Autodesk Inventor part; units mm, degrees
ref_plane "YZ Plane" through (0, 0, 0) normal (1, 0, 0) x (0, 1, 0)
ref_plane "XY Plane" through (0, 0, 0) normal (0, 0, 1) x (1, 0, 0)
ref_plane "Work Plane1" through (0, 0, -11) normal (0, 0, -1) x (-1, 0, 0)
sketch "Sketch1" plane through (0, 0, 0) normal (0, 0, 1) x (1, 0, 0)
  circle A0 centre (0, 0) radius 32
  dimension "d0" = 64
extrude "Extrusion1" add sketch "Sketch1" along normal blind 10
sketch "Sketch2" plane through (0, 0, 10) normal (0, 0, 1) x (1, 0, 0)
  circle A0 centre (0, 0) radius 32
  line L0 (-31.4325, 6) -> (-6, 6)
  line L1 (-6, 6) -> (-6, 31.4325)
  dimension "d3" = 6
extrude "Extrusion2" cut sketch "Sketch2" against normal through all contours L1 L0 A0 picked at (-8.4207, 22.185)
pattern_circular "Circular Pattern1" count 4 over 360 about axis through (0, 0, 0) along (0, 0, 1) of "Extrusion2"
sketch "Sketch3" plane through (0, 0, 10) normal (0, 0, 1) x (1, 0, 0)
  arc A0 (-31.4325, 6) -> (-31.4325, -6) centre (0, 0) ccw
  arc A1 (31.4325, -6) -> (31.4325, 6) centre (0, 0) ccw
  line L0 (-31.749, 4) -> (31.749, 4)
  line L1 (-31.749, -4) -> (31.749, -4)
  dimension "d9" = 8
extrude "Extrusion3" cut sketch "Sketch3" against normal blind 8
pattern_circular "Circular Pattern2" count 2 over 90 about axis through (0, 0, 0) along (0, 0, 1) of "Extrusion3"
sketch "Sketch4" plane through (0, 0, 0) normal (0, 0, -1) x (-1, 0, 0)
  arc A0 (6, 31.4325) -> (-6, 31.4325) centre (0, 0) ccw
  circle A1 centre (0, 0) radius 5
  dimension "d15" = 10
extrude "Extrusion4" add sketch "Sketch4" along normal blind 16
chamfer "Chamfer1" distance 0.5 angle 45 1 edges at (5, 0, -16)
hole "Hole1" at (5, 0, -11) direction (-1, 0, 0) diameter 2 end through all
ref_plane "Work Plane1" through (0, 0, -11) normal (0, 0, -1) x (-1, 0, 0)
properties part number "Cross" material "Steel"
The model under review builds one solid part; all positions refer to its coordinate system, in mm. A direction names the side the tool comes from. Round coordinates to 2 decimals unless told otherwise and drop trailing zeros. Order: outer loops, then holes, each group sorted by start corner. A loop starts at its lowest first (then second) coordinate and runs counter-clockwise, first axis right, second up. Notation, with made-up numbers: (-3.75, 41) -> (50.25, 41) arc R29 ccw to (50.25, 74) -> close; hole circle Ø11 at (48, -23). An arc over 180 degrees is marked (long way). Write item = value, one per line. Start each with the question number.
Item 1: Mouldability with a two-part tool opening along Y and no side actions: class faces 1 (the face through (0, 0, 2)), 2 (the face through (-4, 18, 6)), 3 (the face through (-1.43, 31.97, 1.6)) as released by +Y, released by -Y, zero draft, split by the parting line, or undercut.
Item 2: For faces 4 (the face through (6, -19, 5)), 5 (the face through (6, 19, 5)), 6 (the face through (-4, -18, 6)), 7 (the face through (-3, 5, 0)), 8 (the face through (-6, 19, 5)), list the 3-axis set-ups (+Z, -Z, +X, -X, +Y, -Y) from which the entire face can be reached by the end or side of a thin tool; tool diameter is ignored.
Item 3: For line 1 along X through (y, z) = (-8, 5); line 2 along Y through (x, z) = (-3, -11), list the stretches that pass through material, from the lowest coordinate up.
Item 4: Consider section B-B on z = 7.75. Write out the cut boundary in (x, y).
Item 5: Consider section D-D on x = 26.5. Write out the cut boundary in (y, z), plus the area to 3 significant figures.
Item 6: Consider section C-C on x = 0. Write out the cut boundary in (y, z), plus the area to 3 significant figures.
Item 7: Consider section A-A on y = 0. Write out the cut boundary in (x, z).
Item 8: Clearance check with flat-ended pins moving along their axes: pin 1 Ø11 at (x, z) = (-24, 5) entering from -Y; pin 2 Ø8 at (x, z) = (-23.5, 5) entering from +Y; pin 3 Ø1 at (y, z) = (0.5, -9.5) entering from +X. State where each tip first meets the part, or that it passes through.
Conclusion:
q1.face_1 = undercut
q1.face_2 = zero draft
q1.face_3 = released by +Y
q2.face_4 = +Z, -Z, +X, -Y
q2.face_5 = +Z, -Z, +X, +Y
q2.face_6 = +Z, +Y, -Y
q2.face_7 = -Z
q2.face_8 = +Z, -Z, -X, +Y
q3.line_1 = -6 to -4, 4 to 6
q3.line_2 = -4 to -1, 1 to 4
q4.outline = (-31.75, -4) arc R32 ccw to (-31.43, -6) -> (-6, -6) -> (-6, -31.43) arc R32 ccw to (-4, -31.75) -> (-4, -4) -> close; (-31.75, 4) -> (-4, 4) -> (-4, 31.75) arc R32 ccw to (-6, 31.43) -> (-6, 6) -> (-31.43, 6) arc R32 ccw to start; (4, -31.75) arc R32 ccw to (6, -31.43) -> (6, -6) -> (31.43, -6) arc R32 ccw to (31.75, -4) -> (4, -4) -> close; (4, 4) -> (31.75, 4) arc R32 ccw to (31.43, 6) -> (6, 6) -> (6, 31.43) arc R32 ccw to (4, 31.75) -> close
q5.outline = (-6, 0) -> (6, 0) -> (6, 10) -> (4, 10) -> (4, 2) -> (-4, 2) -> (-4, 10) -> (-6, 10) -> close
q5.area = 56.0 mm2
q6.outline = (-32, 0) -> (-5, 0) -> (-5, -15.5) -> (-4.5, -16) -> (4.5, -16) -> (5, -15.5) -> (5, 0) -> (32, 0) -> (32, 2) -> (-32, 2) -> close; hole circle Ø2 at (0, -11)
q6.area = 285 mm2
q7.outline = (-32, 0) -> (-5, 0) -> (-5, -10) -> (5, -10) -> (5, 0) -> (32, 0) -> (32, 2) -> (-32, 2) -> close; (-5, -15.5) -> (-4.5, -16) -> (4.5, -16) -> (5, -15.5) -> (5, -12) -> (-5, -12) -> close
q8.pin_1 = -6
q8.pin_2 = 6
q8.pin_3 = 5
